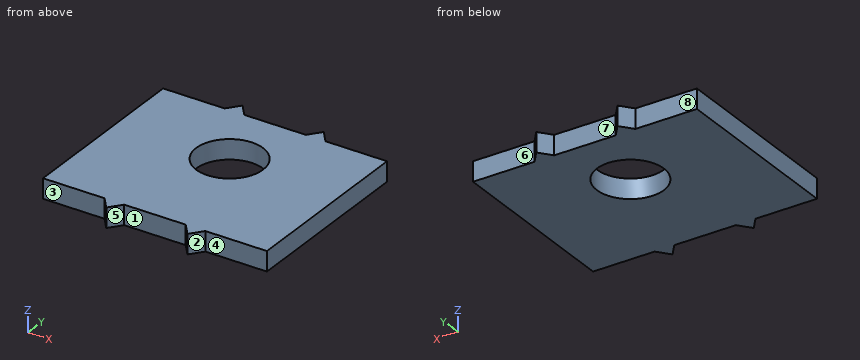
```python
from build123d import *

# Parameters (mm, degrees)
SKETCH1_W        = 45.5
SKETCH1_H        = 37
BASIS_DEPTH      = 4
SKETCH2_R        = 6.8
CAMERA_GAT_DEPTH = 4


with BuildPart() as part:
    # Sketch1 → Basis (new body)
    with BuildSketch(Plane.XY):
        with Locations((22.75, 18.5)):
            Rectangle(SKETCH1_W, SKETCH1_H)
        Polygon((14.5, 39.5), (12.5, 37), (16.5, 37), align=None)
        Polygon((31, 39.5), (29, 37), (33, 37), align=None)
        Polygon((16.5, 0), (12.5, 0), (14.5, -2.5), align=None)
        Polygon((33, 0), (29, 0), (31, -2.5), align=None)
    extrude(amount=BASIS_DEPTH)

    # Sketch2 → Camera gat (cut)
    with BuildSketch(Plane.XY.offset(4)):
        with Locations((22.75, 23)):
            Circle(SKETCH2_R)
    extrude(amount=-CAMERA_GAT_DEPTH, mode=Mode.SUBTRACT)


solid = part.part
```
Check sheet for the modelled part. Datum: model origin and axes. Units: mm. Face numbers are marked on the shaded views. A direction names the side the tool comes from. Give positions to 0.01 mm unless a question says otherwise; leave off trailing zeros. Order: outer loops, then holes, each group sorted by start corner. A loop starts at its lowest first (then second) coordinate and runs counter-clockwise, first axis right, second up. Notation, with made-up numbers: M -37.5,18.25 L -26.5,18.25 A30 ccw -26.5,44.25 Z; hole C 24.25,-39.5 d4. An arc over 180 degrees is marked long. Answer in a Markdown table with one row per item.
1) Cross-section at C-C, the plane z = 2.05. Enter the section's corners in (x, y), plus the area to 3 significant figures.
Filled sheet:
| item | result |
|---|---|
| outline | M 0,0 L 12.5,0 L 14.5,-2.5 L 16.5,0 L 29,0 L 31,-2.5 L 33,0 L 45.5,0 L 45.5,37 L 33,37 L 31,39.5 L 29,37 L 16.5,37 L 14.5,39.5 L 12.5,37 L 0,37 Z; hole C 22.75,23 d13.6 |
| area | 1,560 mm2 |
2) Cross-section at A-A, the plane y = 23. Enter the section's corners in (x, z), plus the area to 3 significant figures.
Filled sheet:
| item | result |
|---|---|
| outline | M 0,0 L 15.95,0 L 15.95,4 L 0,4 Z; M 29.55,0 L 45.5,0 L 45.5,4 L 29.55,4 Z |
| area | 128 mm2 |
3) Gauge pin test, flat ends, axial feed: P1, Ø2, axis at x = 36, z = 2.5, coming from the +Y side; P2, Ø1.2, axis at x = 6.5, z = 2.5, coming from the -Y side; P3, Ø2, axis at x = 14, z = 1.5, coming from the -Y side. Record the tip position at first contact, or that the pin passes through.
Filled sheet:
| item | result |
|---|---|
| P1 | stops at y = 37 |
| P2 | stops at y = 0 |
| P3 | stops at y = -2.5 |
4) Cross-section at B-B, the plane x = 22.75. Enter the section's corners in (y, z), plus the area to 3 significant figures.
Filled sheet:
| item | result |
|---|---|
| outline | M 0,0 L 16.2,0 L 16.2,4 L 0,4 Z; M 29.8,0 L 37,0 L 37,4 L 29.8,4 Z |
| area | 93.6 mm2 |
5) Cross-section at D-D, the plane x = 36. Enter the section's corners in (y, z), plus the area to 3 significant figures.
Filled sheet:
| item | result |
|---|---|
| outline | M 0,0 L 37,0 L 37,4 L 0,4 Z |
| area | 148 mm2 |
6) Thickness scan on L1, parallel to Y at x = 22.75, z = 1.8; L2, parallel to Y at x = 16.5, z = 0.5; L3, parallel to X at y = 28, z = 2.4. Record the ranges inside material, lowest first. Write a range as [from, to].
Filled sheet:
| item | result |
|---|---|
| L1 | y = [0, 16.2], [29.8, 37] |
| L2 | y = [0, 20.32], [25.68, 37] |
| L3 | x = [0, 18.14], [27.36, 45.5] |
7) Release check for a two-part mould opening along X. For the marked faces 1, 2 and 3 record: +X half, -X half, draft (parallel to the pull), parting line (faces both ways), or undercut.
Filled sheet:
| item | result |
|---|---|
| face 1 | undercut |
| face 2 | +X half |
| face 3 | draft |
8) Access from +Z, -Z, +X, -X, +Y, -Y to the whole of each face (thin tool, end or side, straight path). Record for the marked faces 4, 5, 6, 7 and 8.
Filled sheet:
| item | result |
|---|---|
| face 4 | +Z, -Z, +X, -Y |
| face 5 | +Z, -Z, -Y |
| face 6 | +Z, -Z, +X, +Y |
| face 7 | +Z, -Z, +Y |
| face 8 | +Z, -Z, -X, +Y |
